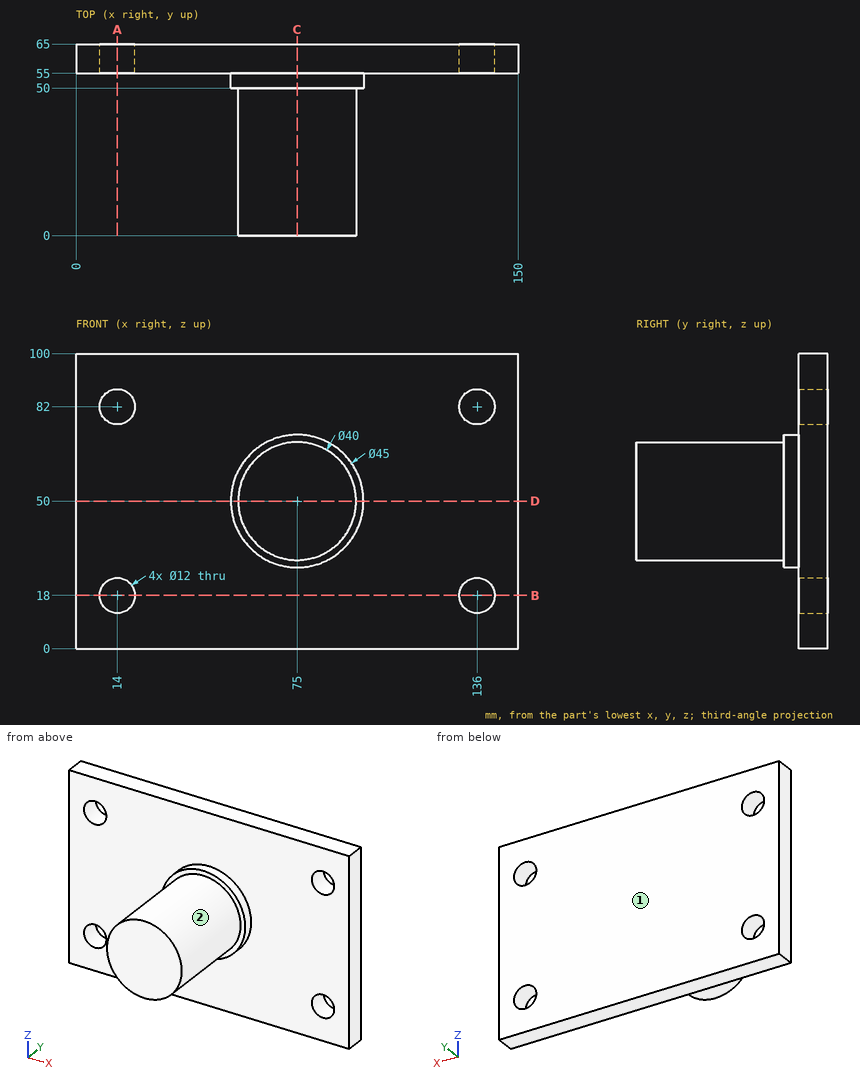
Source: three-view drawing plus pictorial views. Frame: mm from the lowest corner of the part. A direction names the side the tool comes from. Round coordinates to 2 decimals unless told otherwise and drop trailing zeros. Loops run counter-clockwise (first coordinate to the right, second up) from the corner with the lowest first, then second, coordinate; pieces in that order, holes last. Notation, with made-up numbers: M 69.25,61.5 L 128.25,61.5 A16 cw 128.25,91.5 Z; hole C 59,-19 d4. An arc over 180 degrees is marked long. Answer as CSV lines item,"result".
Q1. Cut plane A-A (x = 14). Return the cut outline in (y, z), plus the area to 3 significant figures.
Verdict:
outline,"M 55,0 L 65,0 L 65,12 L 55,12 Z; M 55,24 L 65,24 L 65,76 L 55,76 Z; M 55,88 L 65,88 L 65,100 L 55,100 Z"
area,"760 mm^2"
Q2. Line query: line 1 along Z through (x, y) = (136, 57.25); line 2 along Y through (x, z) = (121, 25); line 3 along X through (y, z) = (7.5, 65). Output: solid intervals per line, ascending.
Verdict:
line 1,"z = 0 to 12, 24 to 76, 88 to 100"
line 2,"y = 55 to 65"
line 3,"x = 61.77 to 88.23"
Q3. Reachability of the marked faces 1 and 2 from +Z, -Z, +X, -X, +Y, -Y: full face, straight path, thin tool, end or side. Return the list, or none.
Verdict:
face 1,"+Z, -Z, +X, -X, +Y"
face 2,"-Y"
Q4. Cut plane D-D (z = 50). Return the cut outline in (x, y), plus the area to 4 significant figures.
Verdict:
outline,"M 0,55 L 52.5,55 L 52.5,50 L 55,50 L 55,0 L 95,0 L 95,50 L 97.5,50 L 97.5,55 L 150,55 L 150,65 L 0,65 Z"
area,"3,725 mm^2"
Q5. Cut plane B-B (z = 18). Return the cut outline in (x, y), plus the area to 3 significant figures.
Verdict:
outline,"M 0,55 L 8,55 L 8,65 L 0,65 Z; M 20,55 L 130,55 L 130,65 L 20,65 Z; M 142,55 L 150,55 L 150,65 L 142,65 Z"
area,"1,260 mm^2"
Q6. Cut plane C-C (x = 75). Return the cut outline in (y, z).
Verdict:
outline,"M 0,30 L 50,30 L 50,27.5 L 55,27.5 L 55,0 L 65,0 L 65,100 L 55,100 L 55,72.5 L 50,72.5 L 50,70 L 0,70 Z"
Q7. Contact query for flat-ended pins moving along their axis: pin 1 (19 mm diameter, centred on x = 14, z = 82, fed in from -Y); pin 2 (6 mm diameter, centred on y = 12.5, z = 31, fed in from +X); pin 3 (6 mm diameter, centred on y = 49.5, z = 62, fed in from -X). Output: stop coordinate, or through.
Verdict:
pin 1,"stops at y = 55"
pin 2,"stops at x = 87"
pin 3,"stops at x = 54.4"
